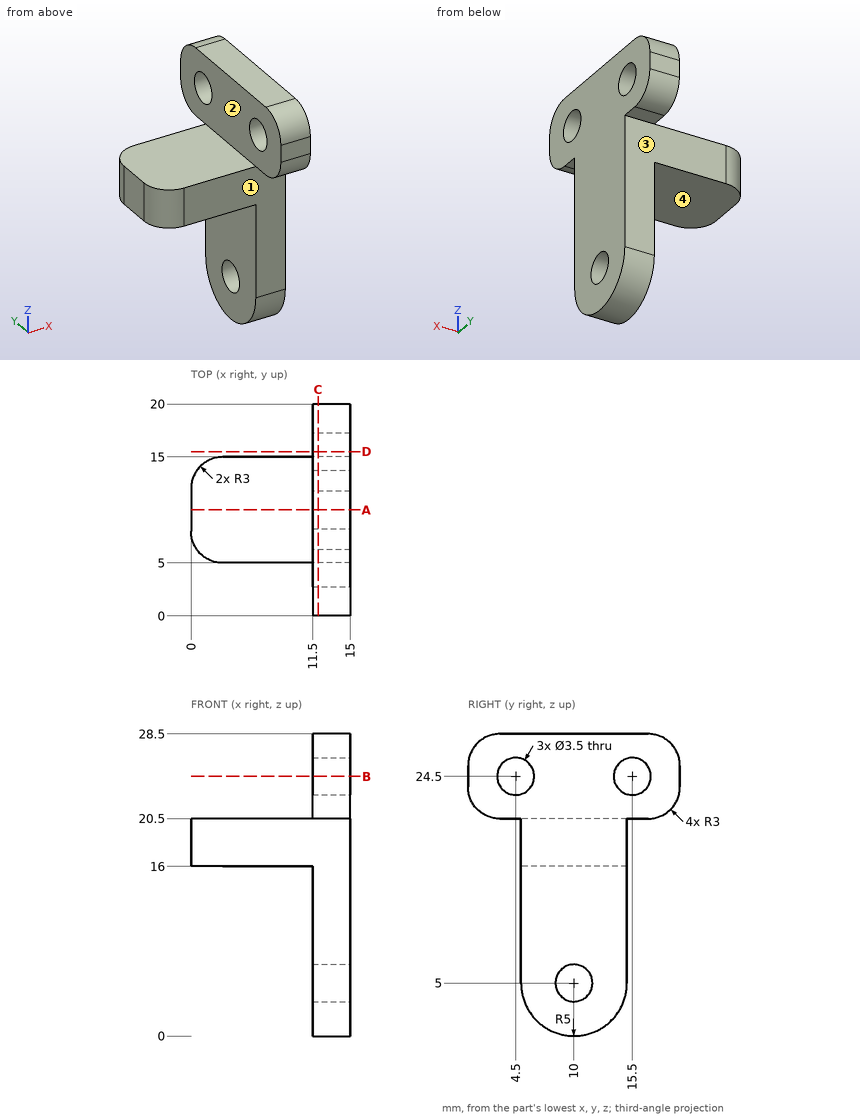
Geometry: see drawing. Coordinates: mm, zero at the bounding-box minimum. A direction names the side the tool comes from. Coordinates: 2 decimals unless noted, no trailing zeros. Write each loop counter-clockwise with the first axis right and the second up, starting at its lowest first coordinate (ties: lowest second). Pieces come first, ordered by that corner, then holes.
1) Material intervals for line 1 along Z through (x, y) = (12.55, 4.5); line 2 along Z through (x, y) = (10.25, 6.75); line 3 along X through (y, z) = (6, 8), sorted ascending.
2) Set-up query: the marked faces 1, 2, 3 and 4. Return all of +Z, -Z, +X, -X, +Y, -Y with unobstructed straight access to the full face (end or side cutting, diameter ignored); none if empty.
3) Section B-B on z = 24.5. Output: boundary loops of the cut face in (x, y), and give its area (3 significant figures).
4) Section D-D on y = 15.5. Output: boundary loops of the cut face in (x, z).
5) Pin query (flat end, axial travel): pin 1 Ø6 at (x, z) = (9.5, 16.5) entering from +Y; pin 2 Ø4 at (x, z) = (4.5, 23.5) entering from +Y; pin 3 Ø2 at (x, y) = (13.5, 3.5) entering from -Z; pin 4 Ø11 at (y, z) = (10, 8) entering from -X. Return the tip coordinate at first contact, or that it passes through.
6) Section A-A on y = 10. Output: boundary loops of the cut face in (x, z), and give its area (3 significant figures).
7) Section C-C on x = 12. Output: boundary loops of the cut face in (y, z), and give its area (3 significant figures).
Check result:
1. line 1: z = 20.5 to 22.75, 26.25 to 28.5
1. line 2: z = 16 to 20.5
1. line 3: x = 11.5 to 15
2. face 1: -Z, +X, -X, -Y
2. face 2: +Z, -X, +Y, -Y
2. face 3: -Z, +X, -X, +Y
2. face 4: -Z, -X, +Y, -Y
3. outline: (11.5, 0) - (15, 0) - (15, 2.75) - (11.5, 2.75) - close; (11.5, 6.25) - (15, 6.25) - (15, 13.75) - (11.5, 13.75) - close; (11.5, 17.25) - (15, 17.25) - (15, 20) - (11.5, 20) - close
3. area: 45.5 mm2
4. outline: (11.5, 20.5) - (15, 20.5) - (15, 22.75) - (11.5, 22.75) - close; (11.5, 26.25) - (15, 26.25) - (15, 28.5) - (11.5, 28.5) - close
5. pin 1: stops at y = 15
5. pin 2: passes through
5. pin 3: stops at z = 20.5
5. pin 4: stops at x = 11.5
6. outline: (0, 16) - (11.5, 16) - (11.5, 6.75) - (15, 6.75) - (15, 28.5) - (11.5, 28.5) - (11.5, 20.5) - (0, 20.5) - close; (11.5, 0) - (15, 0) - (15, 3.25) - (11.5, 3.25) - close
6. area: 139 mm2
7. outline: (0, 23.5) arc R3 ccw to (3, 20.5) - (5, 20.5) - (5, 5) arc R5 ccw to (15, 5) - (15, 20.5) - (17, 20.5) arc R3 ccw to (20, 23.5) - (20, 25.5) arc R3 ccw to (17, 28.5) - (3, 28.5) arc R3 ccw to (0, 25.5) - close; hole circle Ø3.5 at (4.5, 24.5); hole circle Ø3.5 at (10, 5); hole circle Ø3.5 at (15.5, 24.5)
7. area: 318 mm2
